Here's the drawing with two shaded views (mm, measured from the low corner). I have some questions. A direction names the side the tool comes from. Coordinates: 2 decimals unless noted, no trailing zeros. Write each loop counter-clockwise with the first axis right and the second up, starting at its lowest first coordinate (ties: lowest second). Pieces come first, ordered by that corner, then holes.
Item 1: For P1, Ø4, axis at x = 5.5, z = 12.5, coming from the +Y side; P2, Ø1, axis at x = 11.5, y = 8, coming from the -Z side; P3, Ø3, axis at y = 12, z = 24, coming from the -X side; P4, Ø1, axis at y = 10, z = 8.5, coming from the -X side, each with a flat end and sliding along its axis, tell me the tip position at first contact or that it passes through.
Item 2: I want a section at D-D on x = 1. Please give me the cut outline in (y, z), then the cut area to 3 significant figures.
Item 3: I want a section at C-C on z = 24. Please give me the cut outline in (x, y), then the cut area to 3 significant figures.
Item 4: I want a section at A-A on y = 7.5. Please give me the cut outline in (x, z).
Item 5: If I drill on probe 1 along Y at (x, z) = (7.5, 17); probe 2 along Z at (x, y) = (6.75, 2.5); probe 3 along Y at (x, z) = (10, 25.5), over which ranges is the centre line in solid material (lowest first)?
Item 6: Which directions (+Z, -Z, +X, -X, +Y, -Y) give clear straight access to the entire face, cutting with the end or side of a thin tool? Please do the marked faces 1 and 2.
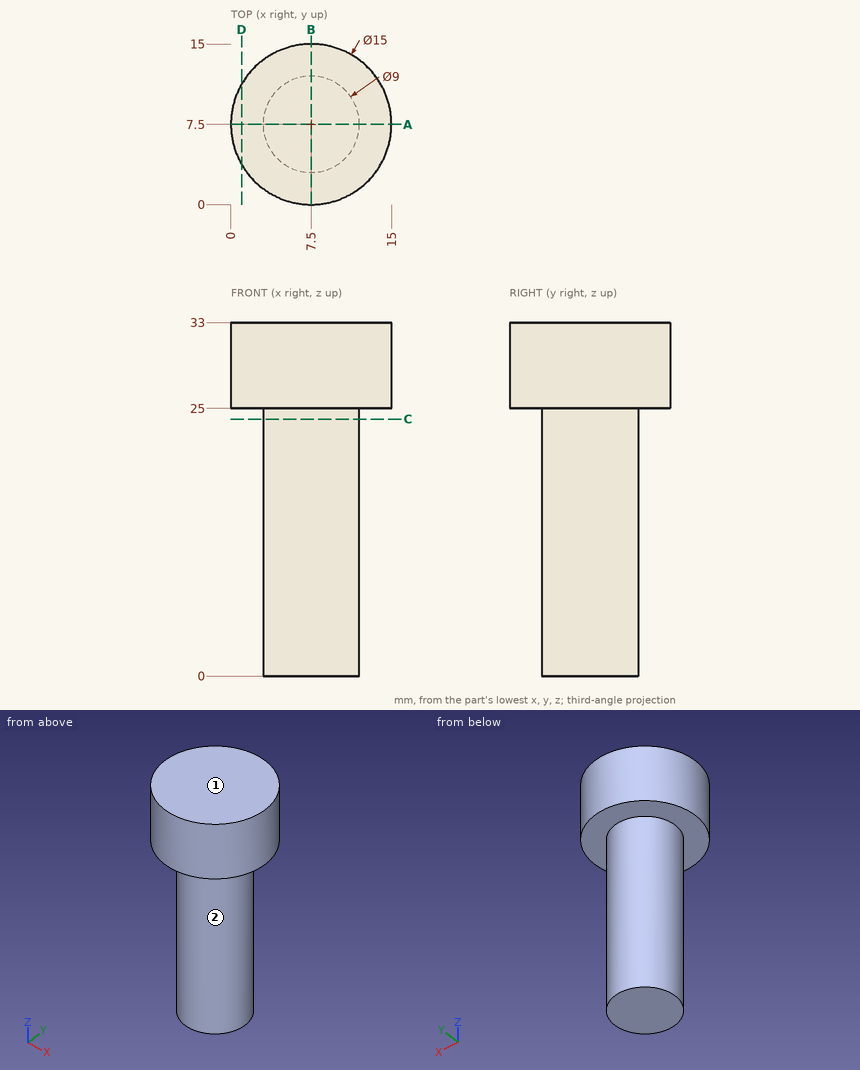
Response values:
1. P1: stops at y = 12
1. P2: stops at z = 0
1. P3: stops at x = 0.81
1. P4: stops at x = 3.47
2. outline: (3.76, 25) - (11.24, 25) - (11.24, 33) - (3.76, 33) - close
2. area: 59.9 mm2
3. outline: circle Ø9 at (7.5, 7.5)
3. area: 63.6 mm2
4. outline: (0, 25) - (3, 25) - (3, 0) - (12, 0) - (12, 25) - (15, 25) - (15, 33) - (0, 33) - close
5. probe 1: y = 3 to 12
5. probe 2: z = 25 to 33
5. probe 3: y = 0.43 to 14.57
6. face 1: +Z, +X, -X, +Y, -Y
6. face 2: -Z
